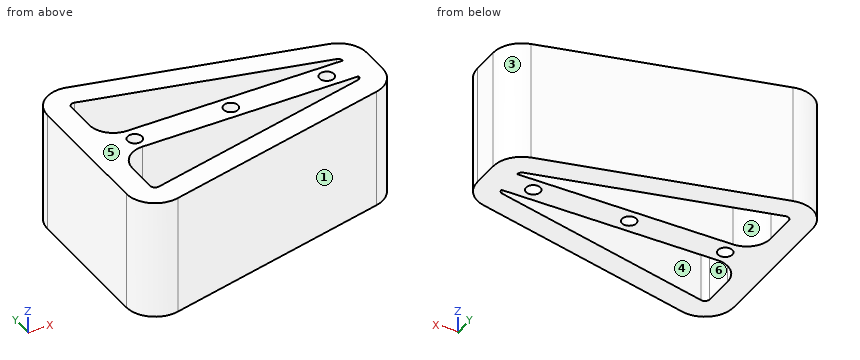
from build123d import *

# Parameters (mm, degrees)
SKETCH1_R           = 1.5
BOSS_EXTRUDE1_DEPTH = 25
FILLET1_R           = 5


with BuildPart() as part:
    # Sketch1 → Boss-Extrude1 (new body)
    with BuildSketch(Plane.XY):
        with BuildLine():
            Line((45, 14.389938011), (45, -14.389938011))
            ThreePointArc((45, -14.389938011), (47.285164876, -19.101625607), (52.4, -20.224318869))
            Line((52.4, -20.224318869), (100.4, -8.70638721))
            ThreePointArc((100.4, -8.70638721), (103.711687596, -6.586841476), (105, -2.872006352))
            Line((105, -2.872006352), (105, 2.872006352))
            ThreePointArc((105, 2.872006352), (103.711687596, 6.586841476), (100.4, 8.70638721))
            Line((100.4, 8.70638721), (52.4, 20.224318869))
            ThreePointArc((52.4, 20.224318869), (47.285164876, 19.101625607), (45, 14.389938011))
        make_face()
        with Locations((75, 0)):
            Circle(SKETCH1_R, mode=Mode.SUBTRACT)
        with Locations((95, 0)):
            Circle(SKETCH1_R, mode=Mode.SUBTRACT)
        with Locations((55, 0)):
            Circle(SKETCH1_R, mode=Mode.SUBTRACT)
        with BuildLine():
            Line((51.233333333, 15.362334821), (99.233333333, 3.844403161))
            ThreePointArc((99.233333333, 3.844403161), (99.785281266, 3.491145539), (100, 2.872006352))
            Line((100, 2.872006352), (50, 2.872006352))
            Line((50, 2.872006352), (50, 14.389938011))
            ThreePointArc((50, 14.389938011), (50.380860813, 15.175219277), (51.233333333, 15.362334821))
        make_face(mode=Mode.SUBTRACT)
        with BuildLine():
            Line((51.233333333, -15.362334821), (99.233333333, -3.844403161))
            ThreePointArc((99.233333333, -3.844403161), (99.785281266, -3.491145539), (100, -2.872006352))
            Line((100, -2.872006352), (50, -2.872006352))
            Line((50, -2.872006352), (50, -14.389938011))
            ThreePointArc((50, -14.389938011), (50.380860813, -15.175219277), (51.233333333, -15.362334821))
        make_face(mode=Mode.SUBTRACT)
    extrude(amount=BOSS_EXTRUDE1_DEPTH)

    # Fillet1
    fillet1_edges = [part.edges().sort_by_distance(p)[0] for p in [
        (50, -2.872006352, 12.5),
        (50, 2.872006352, 12.5),
    ]]
    fillet(fillet1_edges, radius=FILLET1_R)


solid = part.part
Could you check a few things on this model? Use its own coordinates, in mm. Face numbers are marked on the shaded views. A direction names the side the tool comes from. Give positions to 0.01 mm unless a question says otherwise; leave off trailing zeros. Loops run counter-clockwise (first coordinate to the right, second up) from the corner with the lowest first, then second, coordinate; pieces in that order, holes last. Notation, with made-up numbers: M -25,25 L 28,25 A16 ccw 28,52 Z; hole C -10.5,84 d10. An arc over 180 degrees is marked long. Answer as a JSON object with one key per item and string values.
Q1. If I drill on probe 1 along Y at (x, z) = (55, 8.5); probe 2 along Y at (x, z) = (75, 18.75); probe 3 along Y at (x, z) = (84.5, 18.5), over which ranges is the centre line in solid material (lowest first)? Write a range as [from, to].
Values found:
{"probe 1": "y = [-19.6, -14.46], [-2.87, -1.5], [1.5, 2.87], [14.46, 19.6]", "probe 2": "y = [-14.8, -9.66], [-2.87, -1.5], [1.5, 2.87], [9.66, 14.8]", "probe 3": "y = [-12.52, -7.38], [-2.87, 2.87], [7.38, 12.52]"}
Q2. For P1, Ø4, axis at x = 75.5, z = 4.5, coming from the +Y side; P2, Ø8, axis at x = 80.5, z = 4.5, coming from the -Y side; P3, Ø12, axis at x = 69.5, z = 11.5, coming from the -Y side, each with a flat end and sliding along its axis, tell me the tip position at first contact or that it passes through.
Values found:
{"P1": "stops at y = 15.16", "P2": "stops at y = -14.44", "P3": "stops at y = -17.56"}
Q3. Suppose I cut it at B-B, the plane x = 75. List the corners of the cut face in (y, z) for me, plus the area to 3 significant figures.
Values found:
{"outline": "M -14.8,0 L -9.66,0 L -9.66,25 L -14.8,25 Z; M -2.87,0 L -1.5,0 L -1.5,25 L -2.87,25 Z; M 1.5,0 L 2.87,0 L 2.87,25 L 1.5,25 Z; M 9.66,0 L 14.8,0 L 14.8,25 L 9.66,25 Z", "area": "326 mm²"}
Q4. Suppose I cut it at C-C, the plane z = 16. List the corners of the cut face in (x, y) for me.
Values found:
{"outline": "M 45,-14.39 A6 ccw 52.4,-20.22 L 100.4,-8.71 A6 ccw 105,-2.87 L 105,2.87 A6 ccw 100.4,8.71 L 52.4,20.22 A6 ccw 45,14.39 Z; hole M 50,-14.39 A1 ccw 51.23,-15.36 L 99.23,-3.84 A1 ccw 100,-2.87 L 55,-2.87 A5 ccw 50,-7.87 Z; hole M 50,7.87 A5 ccw 55,2.87 L 100,2.87 A1 ccw 99.23,3.84 L 51.23,15.36 A1 ccw 50,14.39 Z; hole C 55,0 d3; hole C 75,0 d3; hole C 95,0 d3"}
Q5. If we mould it in two halves opening along Y, with no side actions, what happens to the marked faces 1, 2, 3 and 4? For each: pulls with the +Y half, pulls with the -Y half, needs draft (parallel to the pull), parting line crosses it, or undercut.
Values found:
{"face 1": "pulls with the -Y half", "face 2": "undercut", "face 3": "pulls with the +Y half", "face 4": "undercut"}
Q6. For the marked faces 5 and 6, which set-ups out of +Z, -Z, +X, -X, +Y, -Y let a thin tool reach every point of the face, with its end or its side?
Values found:
{"face 5": "+Z, +X, -X, +Y, -Y", "face 6": "+Z, -Z"}
Q7. Suppose I cut it at A-A, the plane y = 0. List the corners of the cut face in (x, z) for me, plus the area to 4 significant figures.
Values found:
{"outline": "M 45,0 L 53.5,0 L 53.5,25 L 45,25 Z; M 56.5,0 L 73.5,0 L 73.5,25 L 56.5,25 Z; M 76.5,0 L 93.5,0 L 93.5,25 L 76.5,25 Z; M 96.5,0 L 105,0 L 105,25 L 96.5,25 Z", "area": "1,275 mm²"}
Q8. Suppose I cut it at D-D, the plane y = 6. List the corners of the cut face in (x, z) for me, plus the area to 3 significant figures.
Values found:
{"outline": "M 45,0 L 50.36,0 L 50.36,25 L 45,25 Z; M 90.25,0 L 104.12,0 L 104.12,25 L 90.25,25 Z", "area": "481 mm²"}
